The model under review builds one solid part; all positions refer to its coordinate system, in mm. Give positions to 0.01 mm unless a question says otherwise; leave off trailing zeros. Loops run counter-clockwise (first coordinate to the right, second up) from the corner with the lowest first, then second, coordinate; pieces in that order, holes last. Notation, with made-up numbers: M 70.25,40 L 83.25,40 A20 ccw 83.25,64 Z; hole C -5,-5.75 d11. An arc over 180 degrees is marked long. Return JSON: item names as keys, results as strings.
```python
from build123d import *

# Parameters (mm, degrees)
F0_R     = 12.5
F1_DEPTH = 10
F2_R     = 8.505
F3_DEPTH = 27.2
F4_SIZE2 = 3
F4_SIZE  = 2.5


with BuildPart() as f1:
    # F0 (on Top) → F1 (new body)
    with BuildSketch(Plane.XY):
        Circle(F0_R)
    extrude(amount=F1_DEPTH)

    # F2 (on Top) → F3 (cut)
    with BuildSketch(Plane.XY):
        Circle(F2_R)
    extrude(amount=F3_DEPTH, mode=Mode.SUBTRACT)

    # F4
    f4_edges = [f1.edges().sort_by_distance(p)[0] for p in [
        (12.5, 0, 5),
        (-12.5, 0, 0),
        (-12.5, 0, 10),
    ]]
    chamfer(f4_edges, length=F4_SIZE, length2=F4_SIZE2)


solid = f1.part
```
1) Consider section C-C on z = 8.25. Write out the cut boundary in (x, y) (3 decimals), then the cut area to 3 significant figures.
From the geometry:
{"outline": "C 0,0 d23.2; hole C 0,0 d17.01", "area": "195 mm²"}
2) Consider section A-A on x = 0. Write out the cut boundary in (y, z) (3 decimals), then the cut area to 3 significant figures.
From the geometry:
{"outline": "M -12.5,2.5 L -9.5,0 L -8.505,0 L -8.505,10 L -9.5,10 L -12.5,7.5 Z; M 8.505,0 L 9.5,0 L 12.5,2.5 L 12.5,7.5 L 9.5,10 L 8.505,10 Z", "area": "64.9 mm²"}
3) Consider section D-D on z = 1.5. Write out the cut boundary in (x, y) (3 decimals).
From the geometry:
{"outline": "C 0,0 d22.6; hole C 0,0 d17.01"}
4) The part is to be moulded in two halves that separate along Y. For faces 1 (the face through (-2.2, -8.4, 10)), 2 (the face through (11.923, 3.755, 4.965)), 3 (the face through (-6.749, -5.175, 4.93)), say which applies: released by +Y, released by -Y, zero draft, split by the parting line, or undercut.
From the geometry:
{"face 1": "zero draft", "face 2": "split by the parting line", "face 3": "undercut"}
5) Insertion check: pin 1 (1.5 mm diameter, centred on x = -8.5, z = 8, fed in from -Y); pin 2 (1.5 mm diameter, centred on x = 6.5, z = 3, fed in from +Y); pin 3 (3 mm diameter, centred on x = -6.5, z = 5, fed in from +Y). Each pin has a flat end and moves straight along its axis. Give the tip position at first contact, or say it passes through.
From the geometry:
{"pin 1": "y = -9.65", "pin 2": "y = 11.1", "pin 3": "y = 11.46"}
6) Wall thickness on L1, parallel to Y at x = 0, z = 6 (3 decimals); L2, parallel to X at y = -0.25, z = 2.75; L3, parallel to X at y = 0, z = 2.25 (3 decimals): over which ranges is each line inside the solid? List them lowest first. Write a range as from..to.
From the geometry:
{"L1": "-12.5..-8.505, 8.505..12.5", "L2": "-12.5..-8.5, 8.5..12.5", "L3": "-12.2..-8.505, 8.505..12.2"}
